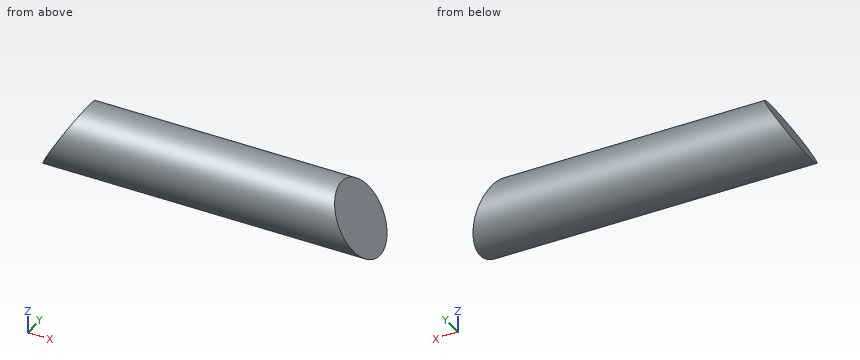
```python
from build123d import *

# Parameters (mm, degrees)
SKETCH_1_R          = 30
EXTRUDE_1_DEPTH     = 150
SKETCH_2_W          = 109.772001157
SKETCH_2_H          = 80.251500104
CUT_EXTRUDE_1_DEPTH = 266.784573674


with BuildPart() as part:
    # 草图1 → 凸台-拉伸1 (new, symmetric)
    with BuildSketch(Plane(origin=(0, 0, 0), x_dir=(0, 0, -1), z_dir=(1, 0, 0))):
        Circle(SKETCH_1_R)
    extrude(amount=EXTRUDE_1_DEPTH, both=True)

    # 草图2 → 切除-拉伸1 (cut, through all)
    with BuildSketch(Plane(origin=(99.240381057, 0, 57.296460718), x_dir=(0, -1, 0), z_dir=(0.866025403784438, 0, 0.500000000000001))):
        with Locations((-4.460929889, 62.152689719)):
            Rectangle(SKETCH_2_W, SKETCH_2_H)
    cut_extrude_1 = extrude(amount=CUT_EXTRUDE_1_DEPTH, mode=Mode.SUBTRACT)

    # 镜向1: 切除-拉伸1 across plane
    add(cut_extrude_1.mirror(Plane(origin=(0, 0, 0), x_dir=(0, 0, 1), z_dir=(1, 0, 0))), mode=Mode.SUBTRACT)


solid = part.part
```
Verification items for the finished model (mm, model axes). Give positions to 0.01 mm unless a question says otherwise; leave off trailing zeros. Order: outer loops, then holes, each group sorted by start corner. A loop starts at its lowest first (then second) coordinate and runs counter-clockwise, first axis right, second up. Notation, with made-up numbers: M -26,-29.5 L -4,-29.5 A23 cw -4,-5.5 Z; hole C -2,4.25 d10. An arc over 180 degrees is marked long. Return JSON: item names as keys, results as strings. Group by question number.
1) Section check B-B on y = 0. Record the cut outline in (x, z), and give its area (3 significant figures).
2) Section check A-A on x = -68. Record the cut outline in (y, z).
3) Section check C-C on z = -26. Record the cut outline in (x, y), and give its area (3 significant figures).
4) Go/stop test with flat-tipped pins: pin 1 Ø10 at (x, y) = (110.5, 9) entering from -Z; pin 2 Ø1 at (x, y) = (-6.5, -19.5) entering from -Z; pin 3 Ø2 at (x, z) = (-40.5, -6) entering from +Y. Record where each tip stops, or that it passes through.
5) Scan lines: line 1 (Z direction, x = -41, y = -0.5); line 2 (Z direction, x = -25.5, y = -3); line 3 (Y direction, x = -74, z = 24). Record each from-to range of solid material in increasing order.
Answer block:
{
 "1": {"outline": "M -149.64,-30 L 149.64,-30 L 115,30 L -115,30 Z", "area": "15,900 mm^2"},
 "2": {"outline": "C 0,0 d60"},
 "3": {"outline": "M -147.33,-14.97 L 147.33,-14.97 L 147.33,14.97 L -147.33,14.97 Z", "area": "8,820 mm^2"},
 "4": {"pin 1": "stops at z = -29.73", "pin 2": "stops at z = -23.22", "pin 3": "stops at y = 29.58"},
 "5": {"line 1": "z = -30 to 30", "line 2": "z = -29.85 to 29.85", "line 3": "y = -18 to 18"}
}
